Autodesk Inventor part; units mm, degrees
ref_plane "Work Plane1" through (29, 0, 0) normal (0, -1, 0) x (1, 0, 0)
ref_plane "YZ Plane" through (0, 0, 0) normal (1, 0, 0) x (0, 1, 0)
ref_plane "XZ Plane" through (0, 0, 0) normal (0, 1, 0) x (-1, 0, 0)
sketch "Sketch1" plane through (0, 0, 0) normal (0, 0, 1) x (1, 0, 0)
  line L0 (-1.1667, 0) -> (100, 0)
  line L1 (100, 0) -> (100, 2.5)
  line L2 (100, 2.5) -> (78, 2.5)
  line L3 (78, 2.5) -> (77.5091, 2.5)
  line L4 (77.5091, 2.5) -> (0, 2.5)
  line L5 (0, 2.5) -> (0, 4.25)
  line L6 (0, 4.25) -> (-5, 4.25)
  line L7 (-5, 4.25) -> (-5, 2.3094)
  line L8 (-5, 2.3094) -> (-2.5, 2.3094)
  line L9 (-2.5, 2.3094) -> (-1.1667, 0)
  line L10 (-26, 0) -> (121, 0)
  line L11 (0, -0.85) -> (0, 5.1)
  line L12 (78, 2.5) -> (0, 2.5) construction
  dimension "d1" = 22
  dimension "d2" = 0.4909
  dimension "d3" = 5
  dimension "d4" = 2.5
  dimension "d5" = 60
  dimension "d6" = 5
  dimension "d7" = 5
  dimension "d8" = 4.6188
  dimension "d9" = 8.5
  dimension "d26" = 100
revolve "Body" add sketch "Sketch1" angle 360 about axis through (-1.1667, 0, 0) along (1, 0, 0)
sketch "Sketch2" plane through (-5, 0, 0) normal (-1, 0, 0) x (0, 0, 1)
  circle A0 centre (0, 0) radius 2.3094
  line L0 (0, -5.95) -> (0, 5.95)
  line L1 (-5.95, 0) -> (5.95, 0)
  line L2 (2.3094, 0) -> (1.1547, -2)
  line L3 (1.1547, -2) -> (-1.1547, -2)
  line L4 (-1.1547, -2) -> (-2.3094, 0)
  line L5 (-2.3094, 0) -> (-1.1547, 2)
  line L6 (-1.1547, 2) -> (1.1547, 2)
  line L7 (1.1547, 2) -> (2.3094, 0)
extrude "Slot" add sketch "Sketch2" against normal up to next contours L7 A0 | A0 L2 | L6 L0 A0 | A0 L0 L3 | L0 L6 A0 | A0 L3 L0 | L4 A0 | A0 L5
fillet "Fillet1" radius 0.5 1 edges at (-5, -4.25, 0)
thread "Thread"
chamfer "Chamfer1" distance 0.4908 distance2 0.4908 1 edges at (100, -2.5, 0) measured on face at (100, 0.2353, -0.3409)
ref_plane "Work Plane1" through (29, 0, 0) normal (0, -1, 0) x (1, 0, 0)
fillet "Fillet2" radius 0.1 1 edges at (0, -2.5, 0)
equation "\"d30\" = R"
equation "\"d17\" = RR"
equation "\"d13\" = GEL"
equation "\"d15\" = -0.5 * SPD + 0.5 * GD"
equation "\"d16\" = GUL"
equation "\"d1\" = GEL"
equation "\"d3\" = KOH"
equation "\"d4\" = INTI"
equation "\"d6\" = GD"
equation "\"d7\" = BDM"
equation "\"d8\" = 1.1547 * SW"
equation "\"d9\" = KOD"
equation "\"d26\" = NLG"
equation "\"GD\" = NND"
equation "\"NLG\" = 100"
equation "\"GEL\" = 22"
equation "\"KOD\" = 8.5"
equation "\"KOH\" = 5"
equation "\"INTI\" = 2.5"
equation "\"GAL\" = 0.61345 * PTC"
equation "\"GUL\" = 0.61345 * PTC"
equation "\"BDM\" = NND"
equation "\"SW\" = 4"
equation "\"RR\" = 0.5"
equation "\"SPD\" = 4.01848"
equation "\"R\" = 0.1"
equation "\"TOA\" = 30deg"
equation "\"THREADDIA\" = 5"
equation "\"PTC\" = 0.8"
equation "\"NND\" = 5"
equation "\"E0\" = 1.155 * SW"
equation "\"GD1\" = THREADDIA - 1.2269 * PTC"
properties part number "ANSI B18.3.1M - M5x0.8 x 100, FSHCSM" material "Steel, Mild"
Part model, mm, in its own coordinate system. A direction names the side the tool comes from. Round coordinates to 2 decimals unless told otherwise and drop trailing zeros. Write each loop counter-clockwise with the first axis right and the second up, starting at its lowest first coordinate (ties: lowest second). Pieces come first, ordered by that corner, then holes. Notation, with made-up numbers: M 5.25,-3.75 L 63.25,-3.75 A24 ccw 63.25,14.25 Z; hole C 43,10 d11. An arc over 180 degrees is marked long. Return JSON: item names as keys, results as strings. Group by question number.
(1) Which spindle directions (+Z, -Z, +X, -X, +Y, -Y) get a long thin tool onto all of the face, cutting with end or side? Do faces 4 (the face through (49.11, -0.54, 2.44)), 5 (the face through (-5, -2, 2)), 6 (the face through (-3.68, 0.99, -1.74)). Say none if no direction does.
(2) Drill centre lines: probe 1 along X at (y, z) = (-2.25, 3); probe 2 along Y at (x, z) = (19.5, 1.5). Where is each one in solid material? Low to high.
(3) Pin check, flat tips, straight feed: pin 1 Ø4 at (x, y) = (45.5, 3) entering from +Z; pin 2 Ø5 at (x, z) = (68.5, -2.5) entering from -Y; pin 3 Ø3 at (y, z) = (-2.5, -2) entering from +X; pin 4 Ø5 at (x, y) = (46.5, 1) entering from -Z. Stop position of each tip, or through.
(4) Two-plate mould, pull along Y, no slides. Class faces 1 (the face through (-2.282, 2.285, -3.584)), 2 (the face through (-3.68, -0.99, 1.74)), 3 (the face through (100, 0, 0)): +Y half, -Y half, draft (parallel to the pull), parting line (faces both ways), or undercut.
(5) Saw through at A-A on x = 72. Write the cut outline in (y, z).
Returned:
{
 "1": {"face 4": "+X", "face 5": "+Z, -Z, -X, +Y, -Y", "face 6": "-X"},
 "2": {"probe 1": "-5 to 0", "probe 2": "-2 to 2"},
 "3": {"pin 1": "z = 2.29", "pin 2": "y = -2.5", "pin 3": "x = 100", "pin 4": "z = -2.5"},
 "4": {"face 1": "parting line", "face 2": "undercut", "face 3": "draft"},
 "5": {"outline": "C 0,0 d5"}
}
